Solid Edge part; units mm, degrees
sketch "Sketch1" plane through (0, 0, 0) normal (0, -1, 0) x (1, 0, 0)
  line L0 (-34, -45.75) -> (34, -45.75)
  line L1 (34, -45.75) -> (34, 45.75)
  line L2 (34, 45.75) -> (-34, 45.75)
  line L3 (-34, 45.75) -> (-34, -45.75)
  dimension "D1" = 34
  dimension "D2" = 34
extrude "Protrusion1" add sketch "Sketch1" against normal blind 12
sketch "Sketch2" plane through (0, 0, 0) normal (0, -1, 0) x (1, 0, 0)
  circle A0 centre (0, -14.75) radius 11.25
  circle A1 centre (-15.5, 0.75) radius 1.7
  circle A2 centre (-15.5, -30.25) radius 1.7
  circle A3 centre (15.5, -30.25) radius 1.7
  circle A4 centre (15.5, 0.75) radius 1.7
extrude "Cutout1" cut sketch "Sketch2" against normal through all
sketch "Sketch3" plane through (0, 0, 0) normal (0, -1, 0) x (1, 0, 0)
  circle A0 centre (7.7782, 36.0282) radius 1.4
  circle A1 centre (7.7782, 20.4718) radius 1.4
  circle A2 centre (-7.7782, 20.4718) radius 1.4
  circle A3 centre (-7.7782, 36.0282) radius 1.4
  circle A4 centre (0, 28.25) radius 6
  dimension "D1" = 7.7782
extrude "Cutout2" cut sketch "Sketch3" against normal through all
sketch "Sketch4" plane through (-34, 6, 0) normal (-1, 0, 0) x (0, 0, -1)
  line L0 (-19.89, -6) -> (45.75, -71.64)
  line L1 (45.75, -71.64) -> (45.75, -6)
  line L2 (45.75, -6) -> (-19.89, -6)
extrude "Extrusionsausprägung_2" add sketch "Sketch4" against normal blind 10
sketch "Sketch5" plane through (-34, 38.82, 0) normal (-1, 0, 0) x (0, 0, -1)
  circle A0 centre (33.7465, 1.4635) radius 1.875
  circle A1 centre (19.6043, 15.6057) radius 1.875
  dimension "D1" = 19.6043
extrude "Extrusionsausschnitt_3" cut sketch "Sketch5" against normal blind 14
sketch "Sketch6" plane through (-34, 38.82, 0) normal (-1, 0, 0) x (0, 0, -1)
  line L0 (45.75, -38.82) -> (-31.89, 38.82)
  line L1 (-31.89, 38.82) -> (-17.75, 38.82)
  line L2 (-17.75, 38.82) -> (45.75, -24.68)
  line L3 (45.75, -24.68) -> (45.75, -38.82)
  dimension "D1" = 31.89
extrude "Extrusionsausprägung_4" add sketch "Sketch6" along normal blind 44
sketch "Sketch7" plane through (-54, 31.75, -14) normal (0, -0.7071068, -0.7071068) x (1, 0, 0)
  circle A0 centre (-14, 10.2613) radius 4
  circle A1 centre (-14, -19.7387) radius 4
extrude "Cutout3" cut sketch "Sketch7" against normal up to next
mirror "Mirror1" [suppressed]
sketch "Sketch8" plane through (-78, 38.82, -6.93) normal (-1, 0, 0) x (0, 0.7071068, -0.7071068)
  line L0 (29.953, 0) -> (42.4264, 12.4734)
extrude "Cutout4" cut sketch "Sketch8" against normal through all material side at (-78, 60.05, -36.93)
mirror "Mirror2" [suppressed]
fillet "Verrundung_1" radius 5 2 edges at (34, 6, -45.75) (-34, 30, -45.75)
chamfer "Fase_1" distance 0.5 angle 45 2 edges at (-34, 23.2143, -17.7293) (-34, 37.3565, -31.8715)
chamfer "Fase_2" distance 0.4 angle 45 4 edges at (-17.2, 0, -30.25) (-17.2, 0, 0.75) (13.8, 0, 0.75) (13.8, 0, -30.25)
chamfer "Fase_3" distance 0.4 angle 45 4 edges at (-9.1782, 0, 20.4718) (-9.1782, 0, 36.0282) (6.3782, 0, 36.0282) (6.3782, 0, 20.4718)
chamfer "Fase_4" distance 2.5 angle 45 2 edges at (-11.25, 0, -14.75) (0, 12, -3.5)
chamfer "Fase_5" distance 1.4 angle 45 2 edges at (-6, 0, 28.25) (0, 12, 34.25)
sketch "Sketch9" plane through (-78, 30, -5.18) normal (-1, 0, 0) x (0, 0.7071068, -0.7071068)
  line L0 (-30.4551, -4.9992) -> (-20.4566, 4.9992)
extrude "Extrusionsausschnitt_8" cut sketch "Sketch9" against normal blind 44 material side at (-78, 11.95, 12.82)
sketch "Sketch10" plane through (-78, 36, -11.18) normal (-1, 0, 0) x (0, 0.7071068, -0.7071068)
  line L0 (-57.2262, -23.285) -> (7.4741, 41.4152)
extrude "Cutout5" cut sketch "Sketch10" against normal through all material side at (-78, 11.95, 0)
sketch "Sketch11" plane through (-51, 12, -12.93) normal (0, -1, 0) x (0, 0, -1)
  circle A0 centre (22.82, 22) radius 1.875
  circle A1 centre (-1.18, 22) radius 1.875
  circle A2 centre (-25.18, 22) radius 1.875
extrude "Cutout6" cut sketch "Sketch11" against normal through all
sketch "Sketch12" plane through (-51, 12, -12.93) normal (0, -1, 0) x (0, 0, -1)
  line L0 (32.82, 27) -> (32.82, 22)
  line L1 (-32.82, 27) -> (32.82, 27)
  line L2 (-32.82, 27) -> (-32.82, 17)
  line L3 (-32.82, 17) -> (-18.68, 17)
  line L4 (-18.68, 17) -> (27.82, 17)
  arc A0 (27.82, 17) -> (32.82, 22) centre (27.82, 22) ccw
extrude "Extrusionsausprägung_6" add sketch "Sketch12" along normal blind 5
sketch "Sketch13" plane through (-29, 7, -12.93) normal (0, -1, 0) x (0, 0, -1)
  circle A0 centre (22.82, 0) radius 1.875
  circle A1 centre (-1.18, 0) radius 1.875
  circle A2 centre (-25.18, 0) radius 1.875
extrude "Cutout7" cut sketch "Sketch13" against normal through all
chamfer "Fase_9" distance 0.5 angle 45 3 edges at (-29, 7, -9.875) (-29, 7, 14.125) (-29, 7, -33.875)
chamfer "Fase_10" distance 0.7 angle 45 4 edges at (-72, 24.4942, -6.7442) (-72, 45.7074, -27.9574) (-68, 55.6058, -23.7158) (-68, 34.3926, -2.5026)
properties material "Nylon, allgemein"
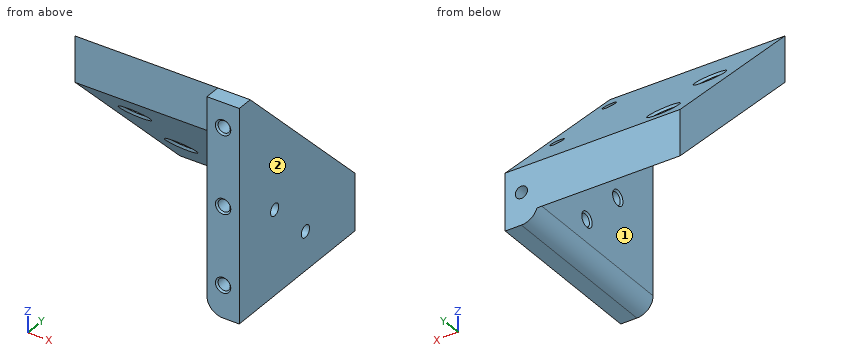
Work out the finished part from the listing and answer in its coordinate system (mm). Face numbers are marked on the shaded views. A direction names the side the tool comes from. Coordinates: 2 decimals unless noted, no trailing zeros. Order: outer loops, then holes, each group sorted by start corner. A loop starts at its lowest first (then second) coordinate and runs counter-clockwise, first axis right, second up. Notation, with made-up numbers: (74.5, 66.25) - (111.5, 66.25) arc R33 ccw to (111.5, 98.25) - close; hole circle Ø9 at (63.5, 46.25). An arc over 180 degrees is marked (long way). Put each result on its own line as item: value. Start each with the question number.
1) Find the intervals of material crossed by line 1 (X direction, y = 11.5, z = 12.25) (3 decimals); line 2 (Z direction, x = -30, y = 13.5); line 3 (X direction, y = 14.25, z = 12.25) (3 decimals), in increasing order. Write a range as from..to.
2) Find section D-D (x = -56.5). Give the vertices of the cut face in (y, z).
3) Find section A-A (z = -11.75). Give the vertices of the cut face in (x, y) (3 decimals).
4) For the marked faces 1 and 2, determine the directions among +Z, -Z, +X, -X, +Y, -Y from which every point of the face is accessible in a straight line to the end or side of a thin tool.
5) Find section C-C (z = 12.25). Give the vertices of the cut face in (x, y) (3 decimals).
6) Flat-ended cylindrical pins translate along their axes: pin 1 (4 mm diameter, centred on x = -47, z = -15, fed in from +Y); pin 2 (3 mm diameter, centred on x = -64.5, z = -31.5, fed in from -Y); pin 3 (5 mm diameter, centred on x = -61, z = 3.5, fed in from +Y); pin 4 (3.5 mm diameter, centred on y = 37.36, z = -33.75, fed in from +X). Find the tip coordinate at first contact, or state that the pin passes through.
7) Find section B-B (y = 14.5). Give the vertices of the cut face in (x, z) (3 decimals).
Results list:
1. line 1: x = -34..-30.875, -27.125..-24
1. line 2: z = -45.65..-37.34, -34.16..-13.34, -10.16..10.66, 13.84..18.39
1. line 3: x = -78..-30.875, -27.125..-24
2. outline: (12, 5.75) - (60, -42.25) - (60, -28.11) - (12, 19.89) - close
3. outline: (-78, 29.5) - (-34, 29.5) - (-34, 7) - (-31.375, 7) - (-30.875, 7.5) - (-30.875, 43.64) - (-78, 43.64) - close; (-27.125, 7.5) - (-26.625, 7) - (-24, 7) - (-24, 43.64) - (-27.125, 43.64) - close
4. face 1: -Z, -X, -Y
4. face 2: +Z, -Z, +X, +Y, -Y
5. outline: (-78, 12) - (-34, 12) - (-34, 7) - (-31.375, 7) - (-30.875, 7.5) - (-30.875, 19.64) - (-78, 19.64) - close; (-27.125, 7.5) - (-26.625, 7) - (-24, 7) - (-24, 19.64) - (-27.125, 19.64) - close
6. pin 1: stops at y = 48.89
6. pin 2: stops at y = 47.76
6. pin 3: stops at y = 30.89
6. pin 4: passes through
7. outline: (-78, 3.25) - (-34, 3.25) - (-34, -40.75) arc R5 ccw to (-29, -45.75) - (-24, -45.75) - (-24, 17.39) - (-78, 17.39) - close; hole circle Ø3.75 at (-29, -35.75); hole circle Ø3.75 at (-29, -11.75); hole circle Ø3.75 at (-29, 12.25)
